Read the model definition and answer for the solid it produces. Units are mm, in the model's axes. Face numbers are marked on the shaded views. A direction names the side the tool comes from. Give positions to 0.01 mm unless a question says otherwise; leave off trailing zeros. Order: outer loops, then holes, each group sorted by start corner. A loop starts at its lowest first (then second) coordinate and runs counter-clockwise, first axis right, second up.
```python
from build123d import *

# Parameters (mm, degrees)
F1_DEPTH = 11.1125
F2_W     = 6.35
F2_H     = 0.5200478494
F2_H_2   = 0.4923428655
F3_DEPTH = 32.54375
F5_DEPTH = 2.38225
F6_W     = 9.525
F6_H     = 4.7625
F7_DEPTH = 3.175


# Not quite as in the source:
# - a feature names something its author has since deleted; it is built from what else it names


with BuildPart() as f1:
    # F0 (on Front) → F1 (new body)
    with BuildSketch(Plane.XZ):
        Polygon((-30.725677704, 46.6747839019), (-42.3673422778, 46.6747839019), (-42.3673422778, 11.7497839019), (-15.3798422778, 11.7497839019), (-15.3798422778, 46.6747839019), align=None)
    extrude(amount=F1_DEPTH)

    # F2 (on face) → F3 (cut)
    with BuildSketch(Plane.XY.offset(46.6747839019)):
        Polygon((-16.9673422778, -9.525), (-16.9673422778, -1.5875), (-20.1423422778, -1.5875), (-40.7925422778, -1.5875), (-40.7925422778, -9.525), (-37.6187860966, -9.525), (-31.2687860966, -9.525), (-26.4923422778, -9.525), (-20.1423422778, -9.525), align=None)
        with Locations((-23.3173422778, -9.7850239247)):
            Rectangle(F2_W, F2_H)
        with Locations((-34.4437860966, -9.7711714327)):
            Rectangle(F2_W, F2_H_2)
    extrude(amount=-F3_DEPTH, mode=Mode.SUBTRACT)

    # F4 (on face) → F5 (cut, through all)
    with BuildSketch(Plane.XY.offset(14.1310339019)):
        with BuildLine():
            ThreePointArc((-34.4437860966, -9.525), (-32.1987220663, -8.5950640303), (-31.2687860966, -6.35))
            ThreePointArc((-31.2687860966, -6.35), (-36.6888501268, -4.1049359697), (-34.4437860966, -9.525))
        make_face()
    extrude(amount=-F5_DEPTH, mode=Mode.SUBTRACT)

    # F6 (on face) → F7 (cut)
    with BuildSketch(Plane.XZ.offset(11.1125)):
        with Locations((-28.8735922778, 44.2935339019)):
            Rectangle(F6_W, F6_H)
    extrude(amount=-F7_DEPTH, mode=Mode.SUBTRACT)


solid = f1.part
```
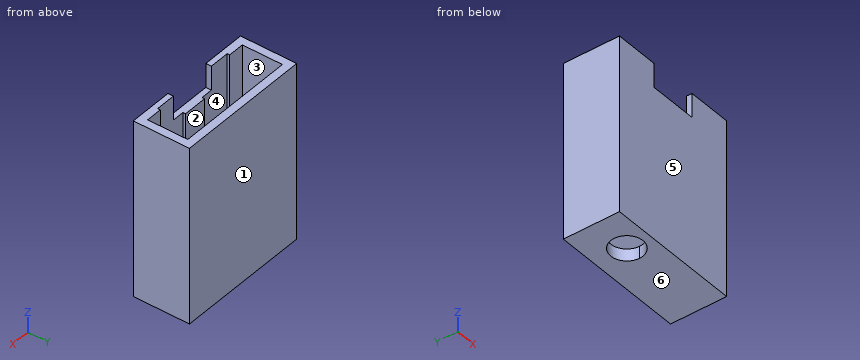
1) The part is cut by section B-B on y = -8. Determine the outline of the cut face in (x, z), and give its area (3 significant figures).
Final values:
outline: (-42.37, 11.75) - (-37.16, 11.75) - (-37.16, 14.13) - (-40.79, 14.13) - (-40.79, 46.67) - (-42.37, 46.67) - close; (-31.73, 11.75) - (-15.38, 11.75) - (-15.38, 46.67) - (-16.97, 46.67) - (-16.97, 14.13) - (-31.73, 14.13) - close
area: 154 mm2
2) The part is cut by section D-D on x = -32.5. Determine the outline of the cut face in (y, z).
Final values:
outline: (-11.11, 11.75) - (-8.86, 11.75) - (-8.86, 14.13) - (-10.02, 14.13) - (-10.02, 41.91) - (-11.11, 41.91) - close; (-3.84, 11.75) - (0, 11.75) - (0, 46.67) - (-1.59, 46.67) - (-1.59, 14.13) - (-3.84, 14.13) - close
3) The part is cut by section A-A on x = -39.25. Determine the outline of the cut face in (y, z) (1 decimal), and give its area (3 significant figures).
Final values:
outline: (-11.1, 11.7) - (0, 11.7) - (0, 46.7) - (-1.6, 46.7) - (-1.6, 14.1) - (-9.5, 14.1) - (-9.5, 46.7) - (-11.1, 46.7) - close
area: 130 mm2
4) A tool of negligible diameter and unlimited length cuts with its end or side. For the marked faces 1 and 2, from which of +Z, -Z, +X, -X, +Y, -Y can it reach the whole face along a straight path? Write none if from no direction.
Final values:
face 1: +Z, -Z, +X, -X, +Y
face 2: +Z
5) Consider L1, parallel to Y at x = -29.25, z = 24 (1 decimal); L2, parallel to X at y = -6.35, z = 13.45; L3, parallel to Y at x = -36, z = 36.5. Determine where each line is inside the solid, lowest interval first.
Final values:
L1: y = -11.1 to -9.5, -1.6 to 0
L2: x = -42.37 to -37.62, -31.27 to -15.38
L3: y = -11.11 to -10.02, -1.59 to 0
6) The part is cut by section C-C on z = 25. Determine the outline of the cut face in (x, y) (1 decimal).
Final values:
outline: (-42.4, -11.1) - (-15.4, -11.1) - (-15.4, 0) - (-42.4, 0) - close; hole (-40.8, -9.5) - (-37.6, -9.5) - (-37.6, -10) - (-31.3, -10) - (-31.3, -9.5) - (-26.5, -9.5) - (-26.5, -10) - (-20.1, -10) - (-20.1, -9.5) - (-17, -9.5) - (-17, -1.6) - (-40.8, -1.6) - close
7) Given pin 1 (1.3 mm diameter, centred on x = -30.5, y = -10.5, fed in from +Z); pin 2 (1 mm diameter, centred on x = -38, z = 15.5, fed in from +Y); pin 3 (4 mm diameter, centred on x = -34.44, y = -6.35, fed in from +Z); pin 4 (1.5 mm diameter, centred on x = -31, y = -7, fed in from +Z), each flat-ended and moving along its own axis, determine where each tip first touches the part or whether it passes through.
Final values:
pin 1: stops at z = 41.91
pin 2: stops at y = 0
pin 3: passes through
pin 4: stops at z = 14.13
8) For a pull along Y with two mould halves and no side action, classify the marked faces 3, 4, 5 and 6 as released by +Y, released by -Y, zero draft, split by the parting line, or undercut.
Final values:
face 3: undercut
face 4: undercut
face 5: released by -Y
face 6: zero draft
